Verification items for the finished model (mm, model axes). A direction names the side the tool comes from. Round coordinates to 2 decimals unless told otherwise and drop trailing zeros. Order: outer loops, then holes, each group sorted by start corner. A loop starts at its lowest first (then second) coordinate and runs counter-clockwise, first axis right, second up. Notation, with made-up numbers: (67, 26.25) -> (103, 26.25) arc R22 cw to (103, 35.25) -> close; hole circle Ø1 at (25.25, 7.25). An arc over 180 degrees is marked (long way). Answer in a Markdown table with one row per item. Add a question column.
```python
from build123d import *

# Parameters (mm, degrees)
BOSS_EXTRUDE1_DEPTH = 4.7625
SKETCH2_R           = 5.08
SKETCH4_R           = 6.604
BOSS_EXTRUDE2_DEPTH = 11.938
SKETCH5_R           = 3.889836973
BOSS_EXTRUDE3_DEPTH = 2.54
SKETCH6_R           = 6.35
BOSS_EXTRUDE4_DEPTH = 1.5875


with BuildPart() as part:
    # Sketch1 → Boss-Extrude1 (new body)
    with BuildSketch(Plane(origin=(0, 0, 0), x_dir=(1, 0, 0), z_dir=(0, 1, 0))):
        Polygon((0, 8.248891971), (-7.14375, 4.124445986), (-7.14375, -4.124445986), (0, -8.248891971), (7.14375, -4.124445986), (7.14375, 4.124445986), align=None)
    extrude(amount=BOSS_EXTRUDE1_DEPTH)

    # Sweep3: sweep along a path in Sketch3
    with BuildLine(Plane(origin=(0, 0, 0), x_dir=(0, 0, -1), z_dir=(1, 0, 0))) as sweep3_path:
        Line((0, 4.7625), (0, 13.843))
        ThreePointArc((0, 13.843), (-1.52509499, 17.52490501), (-5.207, 19.05))
        Line((-5.207, 19.05), (-17.78, 19.05))
    # Sketch2 → Sweep3 (sweep)
    with BuildSketch(Plane(origin=(0, 4.7625, 0), x_dir=(1, 0, 0), z_dir=(0, 1, 0))):
        Circle(SKETCH2_R)
    sweep(path=sweep3_path.line)

    # Sketch4 → Boss-Extrude2 (add)
    with BuildSketch(Plane.XY.offset(17.78)):
        with Locations((0, 19.05)):
            Circle(SKETCH4_R)
    extrude(amount=-BOSS_EXTRUDE2_DEPTH)

    # Sketch5 → Boss-Extrude3 (add)
    with BuildSketch(Plane.XY.offset(17.78)):
        with Locations((0, 19.05)):
            Circle(SKETCH5_R)
    extrude(amount=BOSS_EXTRUDE3_DEPTH)

    # Sketch6 → Boss-Extrude4 (add)
    with BuildSketch(Plane.XY.offset(20.32)):
        with Locations((0, 19.05)):
            Circle(SKETCH6_R)
    extrude(amount=BOSS_EXTRUDE4_DEPTH)


solid = part.part
```
1) Cross-section at B-B, the plane y = 2. Record the boundary of the cut face in (x, z), and give its area (3 significant figures).
2) Cross-section at A-A, the plane x = 5.5. Record the boundary of the cut face in (y, z).
3) Draft check along Y on faces 6 (the face through (-0.84, 15.25, 19.03)), 7 (the face through (2, 14, 5.842)), 8 (the face through (-3.62, 2.35, 6.16)), 9 (the face through (-5, 4.762, 2)). Enter one of: +Y half, -Y half, draft (parallel to the pull), parting line (faces both ways), or undercut.
4) Depth check by flat-ended pin: P1, Ø6.5, axis at x = 2, y = 17, coming from the -Z side; P2, Ø6.5, axis at x = 0, y = 19, coming from the -Z side; P3, Ø5, axis at y = 16, z = 9.5, coming from the -X side. Enter the tip coordinate at first touch or a pass-through.
5) Cross-section at D-D, the plane x = 1. Record the boundary of the cut face in (y, z), and give its area (3 significant figures).
6) Tool access check on faces 1 (the face through (3.522, 2.348, 6.216)), 2 (the face through (-1.1, 14.09, 5.53)), 3 (the face through (-3.522, 2.348, -6.216)), 4 (the face through (-1.432, 12.603, 11.895)), 5 (the face through (-7.144, 2, 0)). Record the directions out of +Z, -Z, +X, -X, +Y, -Y that give a thin tool (end or side, any length) a straight path to the whole face; none if there is none.
7) Cross-section at C-C, the plane z = 12.5. Record the boundary of the cut face in (x, y).
8) Thickness scan on L1, parallel to Z at x = 4, y = 22.5; L2, parallel to X at y = 12.5, z = 0; L3, parallel to Z at x = 2, y = 7.25. Record the ranges inside material, lowest first. Write a range as [from, to].
Results below:
| question | item | result |
|---|---|---|
| 1 | outline | (-7.14, -4.12) -> (0, -8.25) -> (7.14, -4.12) -> (7.14, 4.12) -> (0, 8.25) -> (-7.14, 4.12) -> close |
| 1 | area | 177 mm² |
| 2 | outline | (0, -5.07) -> (4.76, -5.07) -> (4.76, 5.07) -> (0, 5.07) -> close; (15.39, 5.84) -> (22.71, 5.84) -> (22.71, 17.78) -> (15.39, 17.78) -> close; (15.88, 20.32) -> (22.22, 20.32) -> (22.22, 21.91) -> (15.88, 21.91) -> close |
| 3 | face 6 | parting line |
| 3 | face 7 | undercut |
| 3 | face 8 | draft |
| 3 | face 9 | undercut |
| 4 | P1 | z = -5.07 |
| 4 | P2 | z = -4.9 |
| 4 | P3 | x = -6.58 |
| 5 | outline | (0, -7.67) -> (4.76, -7.67) -> (4.76, -4.98) -> (13.84, -4.98) arc R10.19 ccw to (24.03, 5.21) -> (24.03, 5.84) -> (25.58, 5.84) -> (25.58, 17.78) -> (22.81, 17.78) -> (22.81, 20.32) -> (25.32, 20.32) -> (25.32, 21.91) -> (12.78, 21.91) -> (12.78, 20.32) -> (15.29, 20.32) -> (15.29, 17.78) -> (12.52, 17.78) -> (12.52, 5.84) -> (14.07, 5.84) -> (14.07, 5.21) arc R0.23 cw to (13.84, 4.98) -> (4.76, 4.98) -> (4.76, 7.67) -> (0, 7.67) -> close |
| 5 | area | 446 mm² |
| 6 | face 1 | +Z, +X, -Y |
| 6 | face 2 | none |
| 6 | face 3 | -Z, -X, +Y, -Y |
| 6 | face 4 | +Z |
| 6 | face 5 | +Z, -Z, -X, +Y, -Y |
| 7 | outline | circle Ø13.21 at (0, 19.05) |
| 8 | L1 | [5.84, 17.78], [20.32, 21.91] |
| 8 | L2 | [-5.08, 5.08] |
| 8 | L3 | [-4.67, 4.67] |
